CAD build for the part. Positions are in the model's coordinates, mm. Coordinates: 2 decimals unless noted, no trailing zeros. Order: outer loops, then holes, each group sorted by start corner. A loop starts at its lowest first (then second) coordinate and runs counter-clockwise, first axis right, second up. Notation, with made-up numbers: (-29.75, 2) - (-8.75, 2) arc R25 ccw to (-8.75, 38) - close; hole circle Ø4 at (-36, 70). An arc over 180 degrees is marked (long way). Return JSON: item names as keys, results as strings.
from build123d import *

# Parameters (mm, degrees)
SKETCH1_W           = 42
SKETCH1_H           = 48
SKETCH1_R           = 19
SKETCH1_R_2         = 2.5
BOSS_EXTRUDE1_DEPTH = 3
FILLET1_R           = 5


with BuildPart() as part:
    # Sketch1 → Boss-Extrude1 (new body)
    with BuildSketch(Plane.XY):
        Rectangle(SKETCH1_W, SKETCH1_H)
        Circle(SKETCH1_R, mode=Mode.SUBTRACT)
        with Locations((-16, 18.285714286)):
            Circle(SKETCH1_R_2, mode=Mode.SUBTRACT)
        with Locations((16, 18.285714286)):
            Circle(SKETCH1_R_2, mode=Mode.SUBTRACT)
        with Locations((16, -18.285714286)):
            Circle(SKETCH1_R_2, mode=Mode.SUBTRACT)
        with Locations((-16, -18.285714286)):
            Circle(SKETCH1_R_2, mode=Mode.SUBTRACT)
    extrude(amount=BOSS_EXTRUDE1_DEPTH)

    # Fillet1
    fillet1_edges = [part.edges().sort_by_distance(p)[0] for p in [
        (21, -24, 1.5),
        (-21, -24, 1.5),
        (-21, 24, 1.5),
        (21, 24, 1.5),
    ]]
    fillet(fillet1_edges, radius=FILLET1_R)


solid = part.part
Item 1: Drop flat-ended pins along their axis: P1, Ø4, axis at x = 16, y = -18.29, coming from the +Z side; P2, Ø6.5, axis at x = 16, y = 18.29, coming from the +Z side. Give the stop position or say it passes through.
Findings below:
{"P1": "passes through", "P2": "stops at z = 3"}
Item 2: Band-saw the part on B-B, the plane y = 0. List the corners of the cut face in (x, z).
Findings below:
{"outline": "(-21, 0) - (-19, 0) - (-19, 3) - (-21, 3) - close; (19, 0) - (21, 0) - (21, 3) - (19, 3) - close"}
Item 3: Wall check: L1, parallel to Y at x = 0, z = 0.9; L2, parallel to Y at x = -17.5, z = 2; L3, parallel to Y at x = 16, z = 1.65. Give the ranges that are in metal, low to high. Write a range as [from, to].
Findings below:
{"L1": "y = [-24, -19], [19, 24]", "L2": "y = [-23.77, -20.29], [-16.29, -7.4], [7.4, 16.29], [20.29, 23.77]", "L3": "y = [-24, -20.79], [-15.79, -10.25], [10.25, 15.79], [20.79, 24]"}
Item 4: Band-saw the part on A-A, the plane x = 0. List the corners of the cut face in (y, z), then the cut area to 3 significant figures.
Findings below:
{"outline": "(-24, 0) - (-19, 0) - (-19, 3) - (-24, 3) - close; (19, 0) - (24, 0) - (24, 3) - (19, 3) - close", "area": "30.0 mm²"}
Item 5: Band-saw the part on C-C, the plane z = 0.7. List the corners of the cut face in (x, y).
Findings below:
{"outline": "(-21, -19) arc R5 ccw to (-16, -24) - (16, -24) arc R5 ccw to (21, -19) - (21, 19) arc R5 ccw to (16, 24) - (-16, 24) arc R5 ccw to (-21, 19) - close; hole circle Ø38 at (0, 0); hole circle Ø5 at (-16, -18.29); hole circle Ø5 at (-16, 18.29); hole circle Ø5 at (16, -18.29); hole circle Ø5 at (16, 18.29)"}
Item 6: Mould opens along X. For faces 1 (the flat face through (0, -24, 1)), 2 (the cylindrical face through (8.767, -16.856, 1.479)), 3 (the cylindrical face through (-20, 22, 2)) say: released by +X, released by -X, zero draft, split by the parting line, or undercut.
Findings below:
{"face 1": "zero draft", "face 2": "undercut", "face 3": "released by -X"}
